The model under review builds one solid part; all positions refer to its coordinate system, in mm. Face numbers are marked on the shaded views. Round coordinates to 2 decimals unless told otherwise and drop trailing zeros. Loops run counter-clockwise (first coordinate to the right, second up) from the corner with the lowest first, then second, coordinate; pieces in that order, holes last. Notation, with made-up numbers: (-29.5, 78.25) -> (1.5, 78.25) arc R6 ccw to (1.5, 86.25) -> close; hole circle Ø2 at (47, 69.5). An arc over 180 degrees is marked (long way). Write each question's results on one line, items separated by ' | '. Start each with the question number.
Item 1: We need section C-C (y = -28). Give the boundary of the cut face in (x, z), and give its area (3 significant figures).
Item 2: Mouldability with a two-part tool opening along X and no side actions: class the marked faces 1 and 2 as pulls with the +X half, pulls with the -X half, needs draft (parallel to the pull), parting line crosses it, or undercut.
Item 3: We need section D-D (x = 37). Give the boundary of the cut face in (y, z).
Item 4: For L1, parallel to Y at x = -50.8, z = 5; L2, parallel to X at y = 24, z = 6; L3, parallel to X at y = -50, z = 1.25, list the stretches that pass through material, from the lowest coordinate up. Write a range as from..to.
Item 5: Clearance check with a flat-ended pin moving along its axis: pin 1 Ø1.5 at (x, y) = (-25.5, -19) entering from +Z. State where the tip first meets the part, or that it passes through.
Item 6: We need section B-B (y = 50.8). Give the boundary of the cut face in (x, z), and give its area (3 significant figures).
Item 7: We need section A-A (x = -50.8). Give the boundary of the cut face in (y, z), and give its area (3 significant figures).
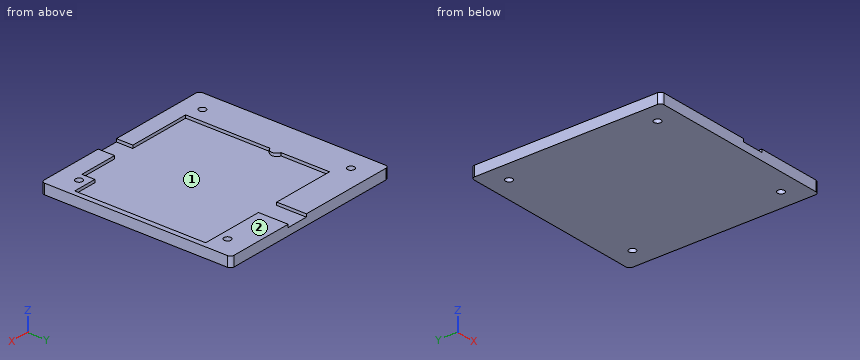
Autodesk Fusion 360 part; units mm, degrees
ref_plane "WorkPlane1" through (0, 0, 7) normal (0, 0, 1) x (1, 0, 0)
sketch "Square Base Plate Sketch" plane through (0, 0, 0) normal (0, 0, 1) x (1, 0, 0)
  line L0 (-65, -65) -> (65, -65)
  line L1 (65, -65) -> (65, 65)
  line L2 (65, 65) -> (-65, 65)
  line L3 (-65, 65) -> (-65, -65)
extrude "Square Base Plate" add sketch "Square Base Plate Sketch" along normal blind 7
fillet "Fillet1" radius 2.5 4 edges at (-65, 65, 3.5) (65, 65, 3.5) (65, -65, 3.5) (-65, -65, 3.5)
sketch "Wafer Nest Pocket Sketch" plane through (0, 0, 7) normal (0, 0, 1) x (1, 0, 0)
  line L0 (-40.523, -53.7567) -> (61.477, -53.7567)
  line L1 (61.477, -53.7567) -> (61.477, 44.704)
  line L2 (61.477, 44.704) -> (-40.523, 44.704)
  line L3 (-40.523, 44.704) -> (-40.523, -53.7567)
extrude "Wafer Nest Pocket" cut sketch "Wafer Nest Pocket Sketch" against normal blind 2
sketch "Front-Center Access Relief Sketch" plane through (0, 0, 7) normal (0, 0, 1) x (1, 0, 0)
  line L0 (2.977, -66) -> (17.977, -66)
  line L1 (17.977, -66) -> (17.977, -50.7567)
  line L2 (17.977, -50.7567) -> (2.977, -50.7567)
  line L3 (2.977, -50.7567) -> (2.977, -66)
extrude "Front-Center Access Relief" cut sketch "Front-Center Access Relief Sketch" against normal blind 2
sketch "Rear-Center Access Relief Sketch" plane through (0, 0, 7) normal (0, 0, 1) x (1, 0, 0)
  line L0 (2.977, 41.704) -> (17.977, 41.704)
  line L1 (17.977, 41.704) -> (17.977, 66)
  line L2 (17.977, 66) -> (2.977, 66)
  line L3 (2.977, 66) -> (2.977, 41.704)
extrude "Rear-Center Access Relief" cut sketch "Rear-Center Access Relief Sketch" against normal blind 2
sketch "X Datum Bump Sketch (165 deg / 9:30)" plane through (0, 0, 7) normal (0, 0, 1) x (1, 0, 0)
  circle A0 centre (-41.683, 7.6802) radius 4
extrude "X Datum Bump (165 deg / 9:30)" add sketch "X Datum Bump Sketch (165 deg / 9:30)" against normal blind 2
sketch "Front-Right Corner Clip (dowel) Sketch" plane through (0, 0, 7) normal (0, 0, 1) x (1, 0, 0)
  line L0 (44.9187, -53.7567) -> (61.477, -53.7567)
  line L1 (61.477, -53.7567) -> (61.477, -44.9187)
  line L2 (61.477, -44.9187) -> (44.9187, -44.9187)
  line L3 (44.9187, -44.9187) -> (44.9187, -53.7567)
extrude "Front-Right Corner Clip (dowel)" add sketch "Front-Right Corner Clip (dowel) Sketch" against normal blind 2
sketch "Outer Front Left Dowel Bore Sketch" plane through (0, 0, 7) normal (0, 0, 1) x (1, 0, 0)
  circle A0 centre (-50.8, -50.8) radius 2.3813
extrude "Outer Front Left Dowel Bore" cut sketch "Outer Front Left Dowel Bore Sketch" against normal blind 7
sketch "Outer Front Right Dowel Bore Sketch" plane through (0, 0, 7) normal (0, 0, 1) x (1, 0, 0)
  circle A0 centre (50.8, -50.8) radius 2.3813
extrude "Outer Front Right Dowel Bore" cut sketch "Outer Front Right Dowel Bore Sketch" against normal blind 7
sketch "Outer Rear Left Dowel Bore Sketch" plane through (0, 0, 7) normal (0, 0, 1) x (1, 0, 0)
  circle A0 centre (-50.8, 50.8) radius 2.3813
extrude "Outer Rear Left Dowel Bore" cut sketch "Outer Rear Left Dowel Bore Sketch" against normal blind 7
sketch "Outer Rear Right Dowel Bore Sketch" plane through (0, 0, 7) normal (0, 0, 1) x (1, 0, 0)
  circle A0 centre (50.8, 50.8) radius 2.3813
extrude "Outer Rear Right Dowel Bore" cut sketch "Outer Rear Right Dowel Bore Sketch" against normal blind 7
equation "gridPitch = 25.4 mm"
equation "indexMove = 50.8 mm"
equation "outerPinPatternSpan = 101.6 mm"
equation "dowelDiameter = 4.7625 mm"
equation "dowelHoleDiameter = 4.7625 mm"
equation "basePlateSize = 130.0 mm"
equation "baseThickness = 7.0 mm"
equation "pocketDepth = 2.0 mm"
equation "nestClearance = 1.0 mm"
equation "filletRadius = 2.5 mm"
equation "primaryFlatClearance = 0.175 mm"
equation "xBumpDiameter = 8.0 mm"
equation "nestReliefWidth = 15.0 mm"
equation "nestOffsetX = 7.29 mm"
equation "nestOffsetY = -4.95 mm"
Here are the results:
1) outline: (-65, 0) -> (65, 0) -> (65, 7) -> (61.48, 7) -> (61.48, 5) -> (-40.52, 5) -> (-40.52, 7) -> (-65, 7) -> close | area: 706 mm2
2) face 1: undercut | face 2: needs draft
3) outline: (-65, 0) -> (65, 0) -> (65, 7) -> (44.7, 7) -> (44.7, 5) -> (-53.76, 5) -> (-53.76, 7) -> (-65, 7) -> close
4) L1: y = -65..-53.18, -48.42..48.42, 53.18..65 | L2: x = -65..-40.52, 61.48..65 | L3: x = -65..-53.04, -48.56..48.56, 53.04..65
5) pin 1: stops at z = 5
6) outline: (-65, 0) -> (-53.18, 0) -> (-53.18, 7) -> (-65, 7) -> close; (-48.42, 0) -> (48.42, 0) -> (48.42, 7) -> (17.98, 7) -> (17.98, 5) -> (2.98, 5) -> (2.98, 7) -> (-48.42, 7) -> close; (53.18, 0) -> (65, 0) -> (65, 7) -> (53.18, 7) -> close | area: 813 mm2
7) outline: (-65, 0) -> (-53.18, 0) -> (-53.18, 7) -> (-65, 7) -> close; (-48.42, 0) -> (48.42, 0) -> (48.42, 7) -> (-48.42, 7) -> close; (53.18, 0) -> (65, 0) -> (65, 7) -> (53.18, 7) -> close | area: 843 mm2
